Job drawing, mm, ordinate dimensions from the low corner. One solid piece. A direction names the side the tool comes from. Round coordinates to 2 decimals unless told otherwise and drop trailing zeros. Loops run counter-clockwise (first coordinate to the right, second up) from the corner with the lowest first, then second, coordinate; pieces in that order, holes last. Notation, with made-up numbers: (-5, 58.5) - (41, 58.5) arc R11 cw to (41, 75.5) - close; hole circle Ø9 at (29, -31.5). An arc over 180 degrees is marked (long way). Answer as CSV lines item,"result". Start each with the question number.
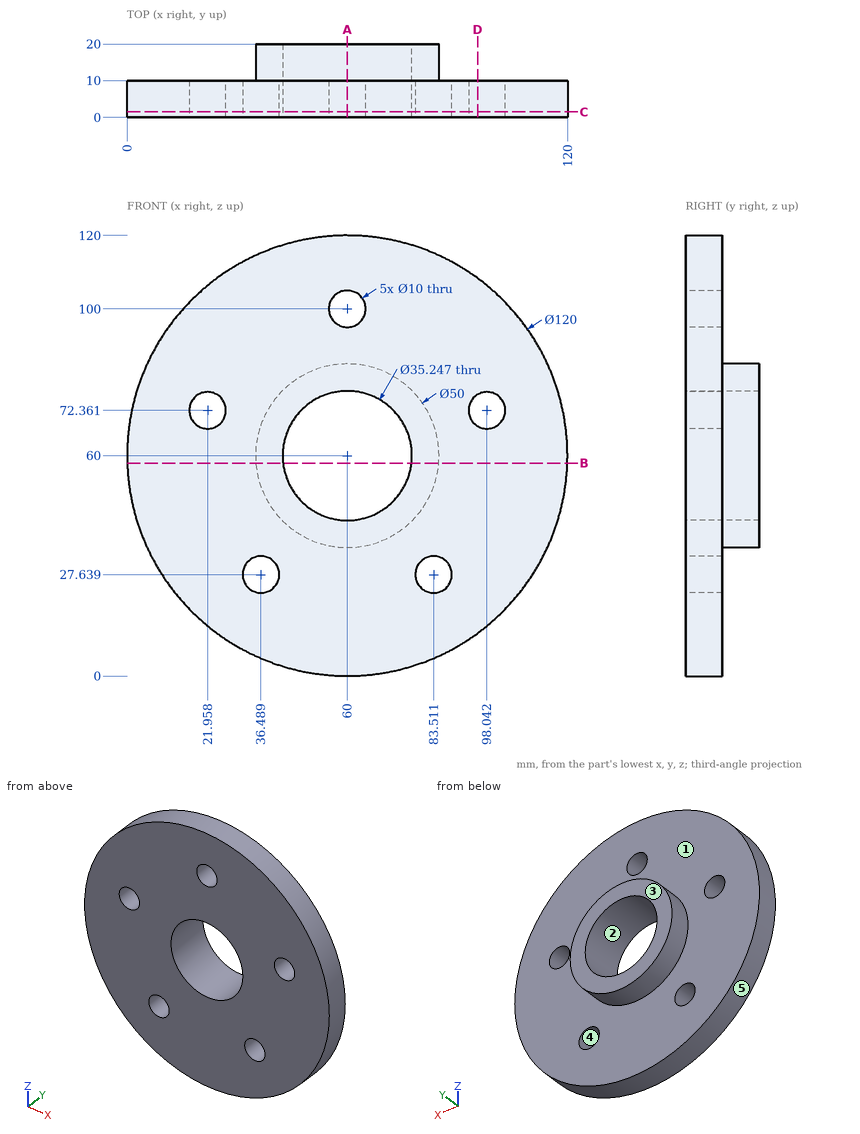
Q1. Band-saw the part on D-D, the plane x = 95.5. List the corners of the cut face in (y, z) (1 decimal).
Q2. Tool access for the marked faces 1 and 2: list every direction of +Z, -Z, +X, -X, +Y, -Y with a clear straight run to the whole face (end or side of a thin tool).
Q3. Two-plate mould, pull along X, no slides. Class the marked faces 3, 4 and 5: released by +X, released by -X, zero draft, split by the parting line, or undercut.
Q4. Band-saw the part on B-B, the plane z = 58. List the corners of the cut face in (x, y).
Q5. Band-saw the part on C-C, the plane y = 1.5. List the corners of the cut face in (x, z).
Q6. Band-saw the part on A-A, the plane x = 60. List the corners of the cut face in (y, z), then the cut area to 3 significant figures.
Q7. Pin check, flat tips, straight feed: pin 1 Ø3 at (y, z) = (9.5, 73.5) entering from -X; pin 2 Ø6 at (x, y) = (63, 16) entering from +Z; pin 3 Ø4 at (y, z) = (10, 15) entering from +X (1 decimal). Stop position of each tip, or through.
Q8. Wall check: probe 1 along Z at (x, y) = (60, 8.5); probe 2 along Y at (x, z) = (72, 19.5); probe 3 along Z at (x, y) = (70, 13.5). Give the ranges that are in metal, low to high. Write a range as [from, to].
Reported:
1,outline,"(0, 11.6) - (10, 11.6) - (10, 68.1) - (0, 68.1) - close; (0, 76.7) - (10, 76.7) - (10, 108.4) - (0, 108.4) - close"
2,face 1,"+Y"
2,face 2,"+Y, -Y"
3,face 3,"zero draft"
3,face 4,"undercut"
3,face 5,"split by the parting line"
4,outline,"(0.03, 0) - (42.49, 0) - (42.49, 20) - (35.08, 20) - (35.08, 10) - (0.03, 10) - close; (77.51, 0) - (119.97, 0) - (119.97, 10) - (84.92, 10) - (84.92, 20) - (77.51, 20) - close"
5,outline,"circle Ø120 at (60, 60); hole circle Ø10 at (21.96, 72.36); hole circle Ø10 at (36.49, 27.64); hole circle Ø35.25 at (60, 60); hole circle Ø10 at (60, 100); hole circle Ø10 at (83.51, 27.64); hole circle Ø10 at (98.04, 72.36)"
6,outline,"(0, 0) - (10, 0) - (10, 35) - (20, 35) - (20, 42.38) - (0, 42.38) - close; (0, 77.62) - (20, 77.62) - (20, 85) - (10, 85) - (10, 95) - (0, 95) - close; (0, 105) - (10, 105) - (10, 120) - (0, 120) - close"
6,area,"895 mm2"
7,pin 1,"stops at x = 1.21"
7,pin 2,"stops at z = 85"
7,pin 3,"stops at x = 101.8"
8,probe 1,"z = [0, 42.38], [77.62, 95], [105, 120]"
8,probe 2,"y = [0, 10]"
8,probe 3,"z = [37.09, 45.49], [74.51, 82.91]"
